Verification items for the finished model (mm, model axes). A direction names the side the tool comes from. Round coordinates to 2 decimals unless told otherwise and drop trailing zeros. Write each loop counter-clockwise with the first axis right and the second up, starting at its lowest first coordinate (ties: lowest second). Pieces come first, ordered by that corner, then holes.
from build123d import *

# Parameters (mm, degrees)
BOSS_EXTRUDE1_DEPTH = 65
SKETCH2_R           = 2.5
CUT_EXTRUDE1_DEPTH  = 10
SKETCH3_W           = 38
SKETCH3_H           = 20
CUT_EXTRUDE2_DEPTH  = 10
SKETCH6_R           = 2.1
CUT_EXTRUDE5_DEPTH  = 6


with BuildPart() as part:
    # Sketch1 → Boss-Extrude1 (new body)
    with BuildSketch(Plane.XY):
        Polygon((0, 0), (0, 35), (5, 35), (5, 5), (40, 5), (40, 0), align=None)
    extrude(amount=BOSS_EXTRUDE1_DEPTH)

    # Sketch2 → Cut-Extrude1 (cut)
    with BuildSketch(Plane(origin=(5, 0, 0), x_dir=(0, 0, -1), z_dir=(1, 0, 0))):
        with Locations((-8, 25.08)):
            Circle(SKETCH2_R)
        with Locations((-8, 14.92)):
            Circle(SKETCH2_R)
        with Locations((-57, 25.08)):
            Circle(SKETCH2_R)
        with Locations((-57, 14.92)):
            Circle(SKETCH2_R)
    extrude(amount=-CUT_EXTRUDE1_DEPTH, mode=Mode.SUBTRACT)

    # Sketch3 → Cut-Extrude2 (cut)
    with BuildSketch(Plane.ZY):
        with Locations((32.5, 20)):
            Rectangle(SKETCH3_W, SKETCH3_H)
    extrude(amount=-CUT_EXTRUDE2_DEPTH, mode=Mode.SUBTRACT)

    # Sketch6 → Cut-Extrude5 (cut, through all)
    with BuildSketch(Plane(origin=(0, 5, 0), x_dir=(1, 0, 0), z_dir=(0, 1, 0))):
        with Locations((36.464466094, -3.535533906)):
            Circle(SKETCH6_R)
        with Locations((8.535533906, -3.535533906)):
            Circle(SKETCH6_R)
        with Locations((36.464466094, -61.464466094)):
            Circle(SKETCH6_R)
        with Locations((8.535533906, -61.464466094)):
            Circle(SKETCH6_R)
    extrude(amount=-CUT_EXTRUDE5_DEPTH, mode=Mode.SUBTRACT)


solid = part.part
Q1. Tool access check on faces 1 (the flat face through (22, 5, 32)), 2 (the flat face through (20, 0, 32)), 3 (the flat face through (2, 20, 13.5)). Record the directions out of +Z, -Z, +X, -X, +Y, -Y that give a thin tool (end or side, any length) a straight path to the whole face; none if there is none.
Recorded:
face 1: +Z, -Z, +X, +Y
face 2: +Z, -Z, +X, -X, -Y
face 3: +X, -X
Q2. Release check for a two-part mould opening along Y. For faces 4 (the flat face through (2, 35, 32)), 5 (the cylindrical face through (2.535, 25.831, 54.615)), 6 (the flat face through (0, 9, 32)) record: released by +Y, released by -Y, zero draft, split by the parting line, or undercut.
Recorded:
face 4: released by +Y
face 5: undercut
face 6: zero draft
Q3. Sectioned sample at B-B (y = 25.08). Enter the section's corners in (x, z).
Recorded:
outline: (0, 0) - (5, 0) - (5, 5.5) - (0, 5.5) - close; (0, 10.5) - (5, 10.5) - (5, 13.5) - (0, 13.5) - close; (0, 51.5) - (5, 51.5) - (5, 54.5) - (0, 54.5) - close; (0, 59.5) - (5, 59.5) - (5, 65) - (0, 65) - close
Q4. Sectioned sample at D-D (y = 3.5). Enter the section's corners in (x, z), plus the area to 3 significant figures.
Recorded:
outline: (0, 0) - (40, 0) - (40, 65) - (0, 65) - close; hole circle Ø4.2 at (8.54, 3.54); hole circle Ø4.2 at (8.54, 61.46); hole circle Ø4.2 at (36.46, 3.54); hole circle Ø4.2 at (36.46, 61.46)
area: 2,540 mm2
Q5. Material ranges on line 1 along Y through (x, z) = (3, 8); line 2 along Z through (x, y) = (1, 25); line 3 along Y through (x, z) = (2, 16), recorded low to high.
Recorded:
line 1: y = 0 to 12.42, 17.42 to 22.58, 27.58 to 35
line 2: z = 0 to 5.5, 10.5 to 13.5, 51.5 to 54.5, 59.5 to 65
line 3: y = 0 to 10, 30 to 35
Q6. Sectioned sample at C-C (z = 46). Enter the section's corners in (x, y), plus the area to 3 significant figures.
Recorded:
outline: (0, 0) - (40, 0) - (40, 5) - (5, 5) - (5, 10) - (0, 10) - close; (0, 30) - (5, 30) - (5, 35) - (0, 35) - close
area: 250 mm2
Q7. Sectioned sample at A-A (z = 57). Enter the section's corners in (x, y).
Recorded:
outline: (0, 0) - (40, 0) - (40, 5) - (5, 5) - (5, 12.42) - (0, 12.42) - close; (0, 17.42) - (5, 17.42) - (5, 22.58) - (0, 22.58) - close; (0, 27.58) - (5, 27.58) - (5, 35) - (0, 35) - close
Q8. Depth check by flat-ended pin: P1, Ø8, axis at y = 25.08, z = 57, coming from the +X side; P2, Ø6.5, axis at x = 36.46, z = 61.46, coming from the +Y side; P3, Ø2, axis at y = 14, z = 56.5, coming from the -X side. Enter the tip coordinate at first touch or a pass-through.
Recorded:
P1: stops at x = 5
P2: stops at y = 5
P3: passes through
